```python
from build123d import *

# Parameters (mm, degrees)
F0_W     = 102.0963229239
F0_H     = 60.8206074685
F1_DEPTH = 25.4
F2_W     = 71.7670321465
F2_H     = 31.1110951006
F3_DEPTH = 25.401
F4_R     = 5.08
F5_SIZE  = 5.08
F7_D     = 6.35
F7_DEPTH = 3.175
F7_TIP   = 1.9077324654


with BuildPart() as f1:
    # F0 (on Front) → F1 (new body)
    with BuildSketch(Plane.XZ):
        with Locations((-13.5734956712, 13.7862348929)):
            Rectangle(F0_W, F0_H)
    extrude(amount=F1_DEPTH)

    # F2 (on face) → F3 (cut, through all)
    with BuildSketch(Plane.XZ.offset(25.4)):
        with Locations((-14.3382139504, 15.5555475503)):
            Rectangle(F2_W, F2_H)
    extrude(amount=-F3_DEPTH, mode=Mode.SUBTRACT)

    # F4
    f4_edges = [f1.edges().sort_by_distance(p)[0] for p in [
        (-50.22173, -12.7, 0),
    ]]
    fillet(f4_edges, radius=F4_R)

    # F5
    f5_edges = [f1.edges().sort_by_distance(p)[0] for p in [
        (21.545302, -12.7, 31.111095),
    ]]
    chamfer(f5_edges, length=F5_SIZE)

    # F7
    with Locations(Plane.XY.offset(44.1965386271)):
        with Locations((-30.4787158966, -7.1609793231)):
            Hole(F7_D / 2, depth=F7_DEPTH)
            with Locations((0, 0, -(F7_DEPTH + F7_TIP / 2))):  # 118° drill point
                Cone(0, F7_D / 2, F7_TIP, mode=Mode.SUBTRACT)


solid = f1.part
```
For this review, take the finished solid that the model builds, in its own axes (mm). A direction names the side the tool comes from. Round coordinates to 2 decimals unless told otherwise and drop trailing zeros. Order: outer loops, then holes, each group sorted by start corner. A loop starts at its lowest first (then second) coordinate and runs counter-clockwise, first axis right, second up.
Q1. Machinability: for faces 1 (the flat face through (-17, -13, 31.111)), 2 (the flat face through (-14, -25.4, -6)), 3 (the cylindrical face through (-32.186, -4.484, 42.587)), which of the approach directions +Z, -Z, +X, -X, +Y, -Y give a long, thin tool a straight path to every point of the face, cutting with its end or side? Answer none if there is none.
Findings below:
face 1: +Y, -Y
face 2: +Z, -Z, +X, -X, -Y
face 3: +Z
Q2. We need section C-C, the plane y = -17.25. Give the boundary of the cut face in (x, z).
Findings below:
outline: (-64.62, -16.62) - (37.47, -16.62) - (37.47, 44.2) - (-64.62, 44.2) - close; hole (-50.22, 5.08) arc R5.08 ccw to (-45.14, 0) - (21.55, 0) - (21.55, 26.03) - (16.47, 31.11) - (-50.22, 31.11) - close
Q3. Wall thickness on line 1 (Z direction, x = -35, y = -4.75); line 2 (X direction, y = -21, z = 11.5); line 3 (Z direction, x = 21, y = -8.75): over which ranges is each line inside the solid? List them lowest first.
Findings below:
line 1: z = -16.62 to 0, 31.11 to 44.2
line 2: x = -64.62 to -50.22, 21.55 to 37.47
line 3: z = -16.62 to 0, 26.58 to 44.2
Q4. Mouldability with a two-part tool opening along Z and no side actions: class faces 4 (the flat face through (37.475, -13, 13)), 5 (the flat face through (-14, -13, -16.624)), 6 (the flat face through (21.545, -13, 13)) as pulls with the +Z half, pulls with the -Z half, needs draft (parallel to the pull), parting line crosses it, or undercut.
Findings below:
face 4: needs draft
face 5: pulls with the -Z half
face 6: undercut
Q5. We need section B-B, the plane x = -1. Give the boundary of the cut face in (y, z).
Findings below:
outline: (-25.4, -16.62) - (0, -16.62) - (0, 0) - (-25.4, 0) - close; (-25.4, 31.11) - (0, 31.11) - (0, 44.2) - (-25.4, 44.2) - close
Q6. We need section A-A, the plane z = 9. Give the boundary of the cut face in (x, y).
Findings below:
outline: (-64.62, -25.4) - (-50.22, -25.4) - (-50.22, 0) - (-64.62, 0) - close; (21.55, -25.4) - (37.47, -25.4) - (37.47, 0) - (21.55, 0) - close
